```python
from build123d import *

# Parameters (mm, degrees)
EXTRUSION1_DEPTH        = 14
ESQUISSE2_W             = 30
ESQUISSE2_H             = 15
EXTRUSION2_DEPTH        = 3
ESQUISSE3_W             = 30
ESQUISSE3_H             = 15
EXTRUSION3_DEPTH        = 3
ESQUISSE4_R             = 3.5
EXTRUSION4_DEPTH        = 5
ENL_V_MAT_EXTRU_1_DEPTH = 18


with BuildPart() as part:
    # Esquisse1 → Extrusion1 (new body)
    with BuildSketch(Plane.XY):
        with BuildLine():
            Line((15, 15), (-15, 15))
            Line((-15, 15), (-15, 0))
            ThreePointArc((-15, 0), (0, -15), (15, 0))
            Line((15, 0), (15, 15))
        make_face()
    extrude(amount=EXTRUSION1_DEPTH)

    # Esquisse2 → Extrusion2 (add)
    with BuildSketch(Plane.XY.offset(14)):
        with Locations((0, 7.5)):
            Rectangle(ESQUISSE2_W, ESQUISSE2_H)
    extrude(amount=EXTRUSION2_DEPTH)

    # Esquisse3 → Extrusion3 (add)
    with BuildSketch(Plane(origin=(0, 0, 0), x_dir=(-1, 0, 0), z_dir=(0, 0, -1))):
        with Locations((0, 7.5)):
            Rectangle(ESQUISSE3_W, ESQUISSE3_H)
    extrude(amount=EXTRUSION3_DEPTH)

    # Esquisse4 → Extrusion4 (add)
    with BuildSketch(Plane(origin=(0, 15, 0), x_dir=(1, 0, 0), z_dir=(0, 1, 0))):
        with Locations(Location((-0.004325278, -7, 0), (0, 0, 90))):
            Circle(ESQUISSE4_R)
    extrude(amount=EXTRUSION4_DEPTH)

    # Esquisse5 → Enlèv. mat.-Extru.1 (cut)
    with BuildSketch(Plane.XY.offset(14)):
        with BuildLine():
            Line((-2.992817477, 0), (2.992817477, 0))
            ThreePointArc((2.992817477, 0), (0, -2.992817477), (-2.992817477, 0))
        make_face()
    extrude(amount=-ENL_V_MAT_EXTRU_1_DEPTH, mode=Mode.SUBTRACT)


solid = part.part
```
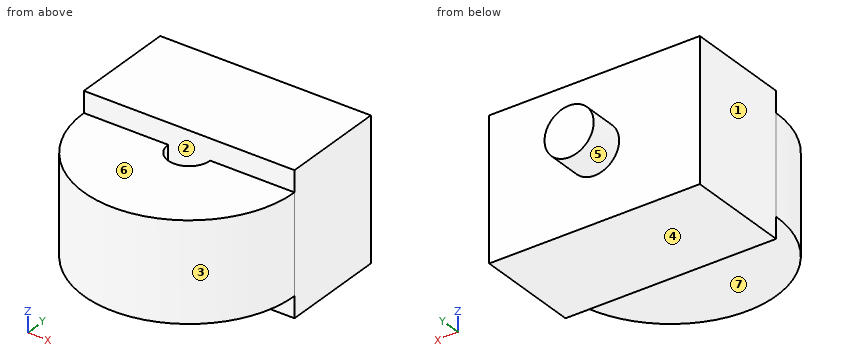
Design review of the part built by this model. Coordinates are the model's own, in mm. Face numbers are marked on the shaded views. A direction names the side the tool comes from. Coordinates: 2 decimals unless noted, no trailing zeros. Order: outer loops, then holes, each group sorted by start corner. A loop starts at its lowest first (then second) coordinate and runs counter-clockwise, first axis right, second up.
1) Take a section at A-A, the plane z = 7. Give the boundary of the cut face in (x, y).
2) Take a section at B-B, the plane x = -11.5. Give the boundary of the cut face in (y, z).
3) Clearance check with flat-ended pins moving along their axes: pin 1 (12 mm diameter, centred on x = 1.5, y = -9.5, fed in from +Z); pin 2 (10 mm diameter, centred on x = -7.5, z = 9.5, fed in from -Y); pin 3 (4 mm diameter, centred on x = 5.5, z = 13, fed in from -Y). State where each tip first meets the part, or that it passes through.
4) For the marked faces 4, 5, 6 and 7, list the 3-axis set-ups (+Z, -Z, +X, -X, +Y, -Y) from which the entire face can be reached by the end or side of a thin tool; tool diameter is ignored.
5) Take a section at D-D, the plane z = 1. Give the boundary of the cut face in (x, y), and give its area (3 significant figures).
6) Mouldability with a two-part tool opening along Y and no side actions: class the marked faces 1, 2 and 3 as +Y half, -Y half, draft (parallel to the pull), parting line (faces both ways), or undercut.
7) Wall thickness on line 1 along Y through (x, z) = (-6.25, -1.5); line 2 along Z through (x, y) = (7, -2.5); line 3 along Y through (x, z) = (-1, 10.75): over which ranges is each line inside the solid? List them lowest first.
8) Take a section at C-C, the plane y = -4.5. Give the boundary of the cut face in (x, z), and give its area (3 significant figures).
Returned:
1. outline: (-15, 0) arc R15 ccw to (15, 0) - (15, 15) - (3.5, 15) - (3.5, 20) - (-3.5, 20) - (-3.5, 15) - (-15, 15) - close; hole (-2.99, 0) arc R2.99 ccw to (2.99, 0) - close
2. outline: (-9.63, 0) - (0, 0) - (0, -3) - (15, -3) - (15, 17) - (0, 17) - (0, 14) - (-9.63, 14) - close
3. pin 1: stops at z = 14
3. pin 2: stops at y = -14.79
3. pin 3: stops at y = -14.59
4. face 4: -Z, +X, -X, +Y, -Y
4. face 5: +Y
4. face 6: +Z, +X, -X, -Y
4. face 7: -Z, +X, -X, -Y
5. outline: (-15, 0) arc R15 ccw to (15, 0) - (15, 15) - (-15, 15) - close; hole (-2.99, 0) arc R2.99 ccw to (2.99, 0) - close
5. area: 789 mm2
6. face 1: draft
6. face 2: undercut
6. face 3: -Y half
7. line 1: y = 0 to 15
7. line 2: z = 0 to 14
7. line 3: y = -14.97 to -2.82, 0 to 15
8. outline: (-14.31, 0) - (14.31, 0) - (14.31, 14) - (-14.31, 14) - close
8. area: 401 mm2
